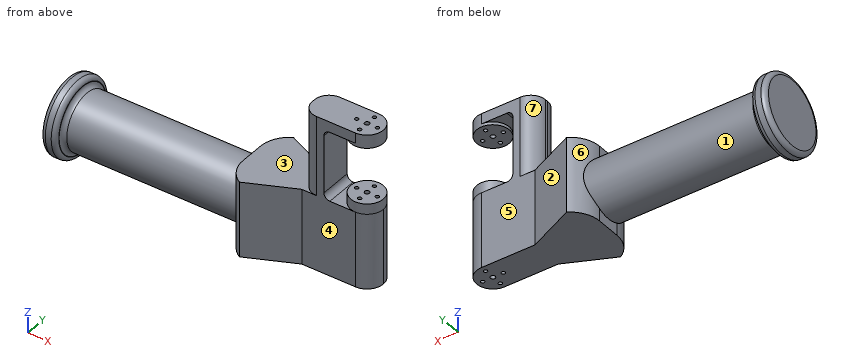
```python
from build123d import *

# Parameters (mm, degrees)
BOSS_EXTRUDE1_DEPTH       = 15
SKETCH2_R                 = 10.97
SKETCH2_R_2               = 1.6
SKETCH2_R_3               = 1.25
BOSS_EXTRUDE2_DEPTH       = 5.89
CUT_EXTRUDE1_START        = -100
SKETCH3_R                 = 1.25
SKETCH3_R_2               = 1.6
CUT_EXTRUDE1_DEPTH        = 100
SKETCH4_W                 = 50
SKETCH4_H                 = 21.94
BOSS_EXTRUDE3_DEPTH       = 49.02
SKETCH9_W                 = 51
SKETCH9_H                 = 51
BOSS_EXTRUDE7_DEPTH       = 10
SKETCH10_R                = 19.05
BOSS_EXTRUDE8_DEPTH       = 114.3
SKETCH11_R                = 25.4
BOSS_EXTRUDE9_DEPTH       = 10
SKETCH12_W                = 15
SKETCH12_H                = 21.94
BOSS_EXTRUDE10_DEPTH      = 30
BOSS_EXTRUDE11_START      = -20.89
SKETCH13_R                = 10.97
SKETCH13_R_2              = 1.6
SKETCH13_R_3              = 1.25
BOSS_EXTRUDE11_DEPTH      = 20.89
CUT_EXTRUDE2_START        = -20.89
SKETCH15_R                = 1.6
SKETCH15_R_2              = 1.25
CUT_EXTRUDE2_DEPTH        = 20.89
SKETCH17_W                = 51
SKETCH17_H                = 51
BOSS_EXTRUDE12_DEPTH      = 79.02
SKETCH18_W                = 30.492655515
SKETCH18_H                = 30.492655514
CUT_EXTRUDE3_DEPTH        = 64
SKETCH19_W                = 15
SKETCH19_H                = 21.94
BOSS_EXTRUDE13_DEPTH      = 29
BOSS_EXTRUDE14_START      = -20.98
SKETCH20_R                = 10.97
SKETCH20_R_2              = 1.6
SKETCH20_R_3              = 1.25
BOSS_EXTRUDE14_DEPTH      = 20.98
CUT_EXTRUDE4_START        = -20.98
SKETCH21_R                = 1.6
SKETCH21_R_2              = 1.25
CUT_EXTRUDE4_DEPTH        = 20.98
SKETCH23_W                = 42.482123656
SKETCH23_H                = 33.824616935
CUT_EXTRUDE6_DEPTH        = 100
FILLET6_R                 = 3
FILLET7_R                 = 3
CUT_EXTRUDE16_DEPTH       = 100
FILLET9_R                 = 20
FILLET10_R                = 20
SKETCH45_W                = 15
SKETCH45_H                = 21.94
BOSS_EXTRUDE19_DEPTH      = 54
SKETCH46_W                = 7
SKETCH46_H                = 21.94
BOSS_EXTRUDE20_DEPTH      = 21.27589
BOSS_EXTRUDE21_DEPTH      = 2
BOSS_EXTRUDE21_DEPTH_BACK = 7
SKETCH47_R                = 10.97
FILLET11_R                = 10
FILLET12_R                = 4
BOSS_EXTRUDE22_START      = 7
SKETCH50_R                = 10.97
BOSS_EXTRUDE22_DEPTH      = 7
CUT_EXTRUDE18_DEPTH       = 149.494915794
CUT_EXTRUDE18_DEPTH_BACK  = 149.494915794
SKETCH51_R                = 1.6
SKETCH51_R_2              = 1.25


with BuildPart() as part:
    # Sketch1 → Boss-Extrude1 (new body)
    with BuildSketch(Plane(origin=(0, 0, 0), x_dir=(0, 0, -1), z_dir=(1, 0, 0))):
        with BuildLine():
            Line((0, 10.97), (80, 10.97))
            Line((80, 10.97), (80, -10.97))
            Line((80, -10.97), (0, -10.97))
            ThreePointArc((0, -10.97), (-10.97, 0), (0, 10.97))
        make_face()
    extrude(amount=BOSS_EXTRUDE1_DEPTH)

    # Sketch2 → Boss-Extrude2 (add)
    with BuildSketch(Plane(origin=(15, 0, 0), x_dir=(0, 0, -1), z_dir=(1, 0, 0))):
        with Locations(Location((0, 0, 0), (0, 0, 270))):
            Circle(SKETCH2_R)
        Circle(SKETCH2_R_2, mode=Mode.SUBTRACT)
        with Locations((0, 6.58)):
            Circle(SKETCH2_R_3, mode=Mode.SUBTRACT)
        with Locations((6.58, 0)):
            Circle(SKETCH2_R_3, mode=Mode.SUBTRACT)
        with Locations((0, -6.58)):
            Circle(SKETCH2_R_3, mode=Mode.SUBTRACT)
        with Locations((-6.58, 0)):
            Circle(SKETCH2_R_3, mode=Mode.SUBTRACT)
    extrude(amount=BOSS_EXTRUDE2_DEPTH)

    # Sketch3 → Cut-Extrude1 (cut)
    with BuildSketch(Plane(origin=(20.89, 0, 0), x_dir=(0, 0, -1), z_dir=(1, 0, 0)).offset(CUT_EXTRUDE1_START)):
        with Locations((0, 6.58)):
            Circle(SKETCH3_R)
        Circle(SKETCH3_R_2)
        with Locations((0, -6.58)):
            Circle(SKETCH3_R)
        with Locations((-6.58, 0)):
            Circle(SKETCH3_R)
        with Locations((6.58, 0)):
            Circle(SKETCH3_R)
    extrude(amount=CUT_EXTRUDE1_DEPTH, mode=Mode.SUBTRACT)

    # Sketch4 → Boss-Extrude3 (add)
    with BuildSketch(Plane(origin=(15, 0, 0), x_dir=(0, 0, -1), z_dir=(1, 0, 0))):
        with Locations((55, 0)):
            Rectangle(SKETCH4_W, SKETCH4_H)
    extrude(amount=BOSS_EXTRUDE3_DEPTH)

    # Sketch9 → Boss-Extrude7 (add)
    with BuildSketch(Plane.ZY):
        with Locations((-54.5, 0)):
            Rectangle(SKETCH9_W, SKETCH9_H)
    extrude(amount=BOSS_EXTRUDE7_DEPTH)

    # Sketch10 → Boss-Extrude8 (add)
    with BuildSketch(Plane.ZY.offset(10)):
        with Locations((-54.5, 0)):
            Circle(SKETCH10_R)
    extrude(amount=BOSS_EXTRUDE8_DEPTH)

    # Sketch11 → Boss-Extrude9 (add)
    with BuildSketch(Plane.ZY.offset(124.3)):
        with Locations((-54.5, 0)):
            Circle(SKETCH11_R)
    extrude(amount=BOSS_EXTRUDE9_DEPTH)

    # Sketch12 → Boss-Extrude10 (add)
    with BuildSketch(Plane.XY.offset(-30)):
        with Locations((56.52, 0)):
            Rectangle(SKETCH12_W, SKETCH12_H)
    extrude(amount=BOSS_EXTRUDE10_DEPTH)

    # Sketch13 → Boss-Extrude11 (add)
    with BuildSketch(Plane(origin=(64.02, 0, 0), x_dir=(0, 0, -1), z_dir=(1, 0, 0)).offset(BOSS_EXTRUDE11_START)):
        with Locations(Location((0, 0, 0), (0, 0, 270))):
            Circle(SKETCH13_R)
        Circle(SKETCH13_R_2, mode=Mode.SUBTRACT)
        with Locations((6.58, 0)):
            Circle(SKETCH13_R_3, mode=Mode.SUBTRACT)
        with Locations((0, 6.58)):
            Circle(SKETCH13_R_3, mode=Mode.SUBTRACT)
        with Locations((0, -6.58)):
            Circle(SKETCH13_R_3, mode=Mode.SUBTRACT)
        with Locations((-6.58, 0)):
            Circle(SKETCH13_R_3, mode=Mode.SUBTRACT)
    extrude(amount=BOSS_EXTRUDE11_DEPTH)

    # Sketch15 → Cut-Extrude2 (cut)
    with BuildSketch(Plane(origin=(64.02, 0, 0), x_dir=(0, 0, -1), z_dir=(1, 0, 0)).offset(CUT_EXTRUDE2_START)):
        Circle(SKETCH15_R)
        with Locations((0, 6.58)):
            Circle(SKETCH15_R_2)
        with Locations((6.58, 0)):
            Circle(SKETCH15_R_2)
        with Locations((0, -6.58)):
            Circle(SKETCH15_R_2)
        with Locations((-6.58, 0)):
            Circle(SKETCH15_R_2)
    extrude(amount=CUT_EXTRUDE2_DEPTH, mode=Mode.SUBTRACT)

    # Sketch17 → Boss-Extrude12 (add)
    with BuildSketch(Plane(origin=(0, 0, 0), x_dir=(0, 0, -1), z_dir=(1, 0, 0))):
        with Locations((54.5, 0)):
            Rectangle(SKETCH17_W, SKETCH17_H)
    extrude(amount=BOSS_EXTRUDE12_DEPTH)

    # Sketch18 → Cut-Extrude3 (cut)
    with BuildSketch(Plane.XY.offset(-29)):
        with Locations((54.797648863, -1.842094242)):
            Rectangle(SKETCH18_W, SKETCH18_H)
    extrude(amount=CUT_EXTRUDE3_DEPTH, mode=Mode.SUBTRACT)

    # Sketch19 → Boss-Extrude13 (add)
    with BuildSketch(Plane.XY.offset(-29)):
        with Locations((71.52, 0)):
            Rectangle(SKETCH19_W, SKETCH19_H)
    extrude(amount=BOSS_EXTRUDE13_DEPTH)

    # Sketch20 → Boss-Extrude14 (add)
    with BuildSketch(Plane(origin=(79.02, 0, 0), x_dir=(0, 0, -1), z_dir=(1, 0, 0)).offset(BOSS_EXTRUDE14_START)):
        with Locations(Location((0, 0, 0), (0, 0, 270))):
            Circle(SKETCH20_R)
        Circle(SKETCH20_R_2, mode=Mode.SUBTRACT)
        with Locations((0, 6.58)):
            Circle(SKETCH20_R_3, mode=Mode.SUBTRACT)
        with Locations((6.58, 0)):
            Circle(SKETCH20_R_3, mode=Mode.SUBTRACT)
        with Locations((0, -6.58)):
            Circle(SKETCH20_R_3, mode=Mode.SUBTRACT)
        with Locations((-6.58, 0)):
            Circle(SKETCH20_R_3, mode=Mode.SUBTRACT)
    extrude(amount=BOSS_EXTRUDE14_DEPTH)

    # Sketch21 → Cut-Extrude4 (cut)
    with BuildSketch(Plane(origin=(79.02, 0, 0), x_dir=(0, 0, -1), z_dir=(1, 0, 0)).offset(CUT_EXTRUDE4_START)):
        Circle(SKETCH21_R)
        with Locations((0, 6.58)):
            Circle(SKETCH21_R_2)
        with Locations((6.58, 0)):
            Circle(SKETCH21_R_2)
        with Locations((0, -6.58)):
            Circle(SKETCH21_R_2)
        with Locations((-6.58, 0)):
            Circle(SKETCH21_R_2)
    extrude(amount=CUT_EXTRUDE4_DEPTH, mode=Mode.SUBTRACT)

    # Sketch23 → Cut-Extrude6 (cut)
    with BuildSketch(Plane(origin=(79.02, 0, 0), x_dir=(0, 0, -1), z_dir=(1, 0, 0))):
        with Locations((7.758938172, -1.322691532)):
            Rectangle(SKETCH23_W, SKETCH23_H)
    extrude(amount=-CUT_EXTRUDE6_DEPTH, mode=Mode.SUBTRACT)

    # Fillet6
    fillet6_edges = [part.edges().sort_by_distance(p)[0] for p in [
        (-124.3, 0, -73.55),
        (-124.3, 0, -79.9),
    ]]
    fillet(fillet6_edges, radius=FILLET6_R)

    # Fillet7
    fillet7_edges = [part.edges().sort_by_distance(p)[0] for p in [
        (-134.3, 0, -79.9),
    ]]
    fillet(fillet7_edges, radius=FILLET7_R)

    # Sketch41 → Cut-Extrude16 (cut)
    with BuildSketch(Plane.XY.offset(-29)):
        with BuildLine():
            Line((79.02, 25.5), (0, 25.5))
            Line((0, 25.5), (31.774109721, 10.97))
            Line((31.774109721, 10.97), (68.05, 10.97))
            ThreePointArc((68.05, 10.97), (75.80696139, 7.75696139), (79.02, 0))
            Line((79.02, 0), (79.02, 25.5))
        make_face()
        with BuildLine():
            Line((31.774109721, -10.97), (0, -25.5))
            Line((0, -25.5), (79.02, -25.5))
            Line((79.02, -25.5), (79.02, 0))
            ThreePointArc((79.02, 0), (75.80696139, -7.75696139), (68.05, -10.97))
            Line((68.05, -10.97), (31.774109721, -10.97))
        make_face()
    extrude(amount=-CUT_EXTRUDE16_DEPTH, mode=Mode.SUBTRACT)

    # Fillet9
    # the kernel refuses this fillet: 20 mm, written as the material it takes off along each edge
    with BuildSketch(Plane(origin=(-10, 25.5, -123.301270189), x_dir=(0, -1, 0), z_dir=(0, 0, 1))) as fillet9_piece_1_section:
        with BuildLine():
            CenterArc((17.320508076, 20), FILLET9_R, 210, 60)
            Line((0, 10), (0, 0))
            Line((0, 0), (17.320508076, 0))
        make_face()
    fillet9_piece_1 = extrude(amount=137.602540378, mode=Mode.PRIVATE)
    fillet9_piece_1 = fillet9_piece_1 - Plane(origin=(-10, 0, -54.5), x_dir=(0, 0, 1), z_dir=(1, 0, 0)) * Cylinder(19.05, 345, mode=Mode.PRIVATE)
    add(fillet9_piece_1, mode=Mode.SUBTRACT)

    # Fillet10
    # the kernel refuses this fillet: 20 mm, written as the material it takes off along each edge
    with BuildSketch(Plane(origin=(-10, -25.5, 14.301270189), x_dir=(0, 1, 0), z_dir=(0, 0, -1))) as fillet10_piece_1_section:
        with BuildLine():
            CenterArc((17.320508076, 20), FILLET10_R, 210, 60)
            Line((0, 10), (0, 0))
            Line((0, 0), (17.320508076, 0))
        make_face()
    fillet10_piece_1 = extrude(amount=137.602540378, mode=Mode.PRIVATE)
    fillet10_piece_1 = fillet10_piece_1 - Plane(origin=(-10, 0, -54.5), x_dir=(0, 0, 1), z_dir=(1, 0, 0)) * Cylinder(19.05, 345, mode=Mode.PRIVATE)
    add(fillet10_piece_1, mode=Mode.SUBTRACT)

    # Sketch45 → Boss-Extrude19 (add)
    with BuildSketch(Plane.XY.offset(-29)):
        with Locations((39.274109721, 0)):
            Rectangle(SKETCH45_W, SKETCH45_H)
    extrude(amount=BOSS_EXTRUDE19_DEPTH)

    # Sketch46 → Boss-Extrude20 (add)
    with BuildSketch(Plane(origin=(46.774109721, 0, 0), x_dir=(0, 0, -1), z_dir=(1, 0, 0))):
        with Locations((-21.5, 0)):
            Rectangle(SKETCH46_W, SKETCH46_H)
    extrude(amount=BOSS_EXTRUDE20_DEPTH)

    # Sketch47 → Boss-Extrude21 (add, two sides: drawn at the far end of the back side and taken through both)
    with BuildSketch(Plane(origin=(0, 0, 18), x_dir=(-1, 0, 0), z_dir=(0, 0, -1)).offset(-BOSS_EXTRUDE21_DEPTH_BACK)):
        with Locations(Location((-68.05, 0, 0), (0, 0, 90))):
            Circle(SKETCH47_R)
    extrude(amount=BOSS_EXTRUDE21_DEPTH + BOSS_EXTRUDE21_DEPTH_BACK)

    # Fillet11
    fillet11_edges = [part.edges().sort_by_distance(p)[0] for p in [
        (31.774109721, 10.97, -2),
        (31.774109721, -10.97, -2),
    ]]
    fillet(fillet11_edges, radius=FILLET11_R)

    # Fillet12
    fillet12_edges = [part.edges().sort_by_distance(p)[0] for p in [
        (46.774109721, 0, -29),
        (46.774109721, 0, 18),
    ]]
    fillet(fillet12_edges, radius=FILLET12_R)

    # Sketch50 → Boss-Extrude22 (add)
    with BuildSketch(Plane.XY.offset(-29).offset(BOSS_EXTRUDE22_START)):
        with Locations((68.05, 0)):
            Circle(SKETCH50_R)
    extrude(amount=-BOSS_EXTRUDE22_DEPTH)

    # Sketch51 → Cut-Extrude18 (cut, two sides: drawn at the far end of the back side and taken through both)
    with BuildSketch(Plane.XY.offset(-22).offset(-CUT_EXTRUDE18_DEPTH_BACK)):
        with Locations((68.05, 0)):
            Circle(SKETCH51_R)
        with Locations((68.05, 7)):
            Circle(SKETCH51_R_2)
        with Locations((75.05, 0)):
            Circle(SKETCH51_R_2)
        with Locations((68.05, -7)):
            Circle(SKETCH51_R_2)
        with Locations((61.05, 0)):
            Circle(SKETCH51_R_2)
    extrude(amount=CUT_EXTRUDE18_DEPTH + CUT_EXTRUDE18_DEPTH_BACK, mode=Mode.SUBTRACT)


solid = part.part
```
Can you work these out from the model? Positions are in its coordinate system, mm. Face numbers are marked on the shaded views. A direction names the side the tool comes from. Coordinates: 2 decimals unless noted, no trailing zeros. Order: outer loops, then holes, each group sorted by start corner. A loop starts at its lowest first (then second) coordinate and runs counter-clockwise, first axis right, second up.
1. Thinking about a two-plate mould opening in X: for the marked faces 1, 2 and 3, which applies, +X half, -X half, draft (parallel to the pull), parting line (faces both ways), or undercut?
2. I need wall thicknesses on line 1 (X direction, y = 0, z = 20); line 2 (Y direction, x = 68, z = 21); line 3 (Y direction, x = 61, z = -36). Which ranges of each line are inside material? Lowest first, please.
3. If we section it at C-C (z = -13): Please give me the cut outline in (x, y).
4. If we section it at A-A (z = -54.5): Please give me the cut outline in (x, y).
5. I'm going to push flat-ended pins straight in: pin 1 (1 mm diameter, centred on y = -0.5, z = 6, fed in from -X); pin 2 (10 mm diameter, centred on x = -16, y = 5.5, fed in from -Z); pin 3 (1 mm diameter, centred on x = -62, y = 17, fed in from +Z). Where does each tip first touch, or does it pass through?
6. For the marked faces 4, 5, 6 and 7, which set-ups out of +Z, -Z, +X, -X, +Y, -Y let a thin tool reach every point of the face, with its end or its side?
7. If we section it at B-B (x = 34): Please give me the cut outline in (y, z).
8. If we section it at D-D (x = -114.5): Please give me the cut outline in (y, z).
Entries:
1. face 1: undercut
1. face 2: +X half
1. face 3: draft
2. line 1: x = 31.77 to 59.8, 62.3 to 66.45, 69.65 to 73.8, 76.3 to 79.02
2. line 2: y = -10.97 to -8.25, -5.75 to -1.6, 1.6 to 5.75, 8.25 to 10.97
2. line 3: y = -10.97 to -1.25, 1.25 to 10.97
3. outline: (31.77, -0.97) arc R10 ccw to (41.77, -10.97) - (46.77, -10.97) - (46.77, 10.97) - (41.77, 10.97) arc R10 ccw to (31.77, 0.97) - close
4. outline: (-134.3, -22.4) arc R3 ccw to (-131.3, -25.4) - (-127.3, -25.4) arc R3 ccw to (-124.3, -22.4) - (-124.3, -22.05) arc R3 cw to (-121.3, -19.05) - (-6.79, -19.05) arc R20 ccw to (0, -25.5) - (31.77, -10.97) - (68.05, -10.97) arc R10.97 ccw to (68.05, 10.97) - (31.77, 10.97) - (0, 25.5) arc R20 ccw to (-6.79, 19.05) - (-121.3, 19.05) arc R3 cw to (-124.3, 22.05) - (-124.3, 22.4) arc R3 ccw to (-127.3, 25.4) - (-131.3, 25.4) arc R3 ccw to (-134.3, 22.4) - close; hole circle Ø2.5 at (61.05, 0); hole circle Ø3.2 at (68.05, 0); hole circle Ø2.5 at (68.05, -7); hole circle Ø2.5 at (68.05, 7); hole circle Ø2.5 at (75.05, 0)
5. pin 1: stops at x = 31.77
5. pin 2: stops at z = -73.54
5. pin 3: stops at z = -44.98
6. face 4: +Z, -Z, +X, -Y
6. face 5: +Z, -Z, +X, +Y
6. face 6: +Y
6. face 7: +Z, -X, +Y
7. outline: (-10.97, -80) - (10.97, -80) - (10.97, -29) - (7.26, -29) - (7.26, 25) - (-7.26, 25) - (-7.26, -29) - (-10.97, -29) - close
8. outline: circle Ø38.1 at (0, -54.5)
